Build history of the part. All positions in model axes, mm. A direction names the side the tool comes from. Round coordinates to 2 decimals unless told otherwise and drop trailing zeros. Loops run counter-clockwise (first coordinate to the right, second up) from the corner with the lowest first, then second, coordinate; pieces in that order, holes last. Notation, with made-up numbers: M 2.5,43 L 11.5,43 A33 ccw 11.5,71 Z; hole C -26.75,-0.75 d2. An arc over 180 degrees is marked long. Write each question's results on one line, items separated by ' | '. Start each with the question number.
```python
from build123d import *

# Parameters (mm, degrees)
F0_R     = 63.5
F0_R_2   = 6.35
F1_DEPTH = 12.7
F0_W     = 12.7
F0_H     = 50.8
F2_DEPTH = 127
F0_W_2   = 25.4
F3_DEPTH = 25.4
F4_R     = 9.525
F5_DEPTH = 254
F6_R     = 3.81


with BuildPart() as f1:
    # F0 (on Front) → F1 (new body)
    with BuildSketch(Plane.XZ):
        Circle(F0_R)
        with Locations((0, -44.45)):
            Circle(F0_R_2, mode=Mode.SUBTRACT)
        with Locations((-44.45, 0)):
            Circle(F0_R_2, mode=Mode.SUBTRACT)
        Polygon((-25.4, -25.4), (-25.4, 25.4), (-12.7, 25.4), (12.7, 25.4), (25.4, 25.4), (25.4, -25.4), (12.7, -25.4), (-12.7, -25.4), align=None, mode=Mode.SUBTRACT)
        with Locations((44.45, 0)):
            Circle(F0_R_2, mode=Mode.SUBTRACT)
        with Locations((0, 44.45)):
            Circle(F0_R_2, mode=Mode.SUBTRACT)
    extrude(amount=F1_DEPTH)

    # F0 (on Front) → F2 (join)
    with BuildSketch(Plane.XZ):
        with Locations((-19.05, 0)):
            Rectangle(F0_W, F0_H)
        with Locations((19.05, 0)):
            Rectangle(F0_W, F0_H)
    extrude(amount=F2_DEPTH)

    # F0 (on Front) → F3 (join)
    with BuildSketch(Plane.XZ):
        Rectangle(F0_W_2, F0_H)
    extrude(amount=F3_DEPTH)

    # F4 (on face) → F5 (cut)
    with BuildSketch(Plane.YZ.offset(25.4)):
        with BuildLine():
            Line((-127, -25.4), (-63.5, -25.4))
            ThreePointArc((-63.5, -25.4), (-88.9, 0), (-63.5, 25.4))
            Line((-63.5, 25.4), (-127, 25.4))
            Line((-127, 25.4), (-127, -25.4))
        make_face()
        with Locations((-63.5, 0)):
            Circle(F4_R)
    extrude(amount=-F5_DEPTH, mode=Mode.SUBTRACT)

    # F6
    f6_edges = [f1.edges().sort_by_distance(p)[0] for p in [
        (0, -12.7, 25.4),
        (25.4, -12.7, 0),
        (0, -12.7, -25.4),
        (-25.4, -12.7, 0),
    ]]
    fillet(f6_edges, radius=F6_R)


solid = f1.part
```
Item 1: Saw through at C-C, the plane z = -44.45. Give the cut face in (x, y), then the cut area to 3 significant figures.
Item 2: Saw through at A-A, the plane x = 0. Give the cut face in (y, z).
Item 3: Saw through at B-B, the plane z = 0. State how many separate pieces and enclosed holes the cut face has, then the cut area to 3 significant figures.
Item 4: Drill centre lines: line 1 along X through (y, z) = (-31.5, 9.5); line 2 along Z through (x, y) = (-16, -63); line 3 along Y through (x, z) = (23, 32). Where is each one in solid material? Low to high. Write a range as [from, to].
Item 5: Tool access for faces 1 (the flat face through (25.4, -52, 0)), 2 (the flat face through (0, -24, 25.4)), 3 (the flat face through (41, -12.7, -13)): list every direction of +Z, -Z, +X, -X, +Y, -Y with a clear straight run to the whole face (end or side of a thin tool).
Item 6: Mould opens along X. For faces 4 (the cylindrical face through (0.409, -13.786, 26.546)), 5 (the cylindrical face through (-0.827, -6.261, 50.746)), 6 (the cylindrical face through (26.546, -13.786, -0.409)), 7 (the flat face through (-25.4, -52, 0)) say: released by +X, released by -X, zero draft, split by the parting line, or undercut.
Item 7: Saw through at D-D, the plane y = -67. Give the cut face in (x, z), then the cut area to 3 significant figures.
Item 8: Drop flat-ended pins along their axis: pin 1 (25 mm diameter, centred on y = -63.5, z = 0, fed in from +X); pin 2 (10 mm diameter, centred on x = -44.45, z = 0, fed in from -Y); pin 3 (10 mm diameter, centred on x = -38.5, z = 22, fed in from -Y); pin 4 (14 mm diameter, centred on x = 1, y = -31, fed in from +Z). Give the stop position or say it passes through.
Working result:
1) outline: M -45.35,-12.7 L -6.35,-12.7 L -6.35,0 L -45.35,0 Z; M 6.35,-12.7 L 45.35,-12.7 L 45.35,0 L 6.35,0 Z | area: 991 mm²
2) outline: M -25.4,-25.4 L -16.51,-25.4 A3.81 cw -12.7,-29.21 L -12.7,-38.1 L 0,-38.1 L 0,38.1 L -12.7,38.1 L -12.7,29.21 A3.81 cw -16.51,25.4 L -25.4,25.4 Z; M -12.7,-63.5 L 0,-63.5 L 0,-50.8 L -12.7,-50.8 Z; M -12.7,50.8 L 0,50.8 L 0,63.5 L -12.7,63.5 Z
3) separate pieces: 5 | enclosed holes: 0 | area: 3,070 mm²
4) line 1: x = [-25.4, -12.7], [12.7, 25.4] | line 2: z = [-25.4, -9.51], [9.51, 25.4] | line 3: y = [-12.7, 0]
5) face 1: +Z, -Z, +X, -Y | face 2: +Z, +X, -X, -Y | face 3: -Y
6) face 4: zero draft | face 5: undercut | face 6: released by +X | face 7: released by -X
7) outline: M -25.4,-25.16 L -12.7,-25.16 L -12.7,-8.86 L -25.4,-8.86 Z; M -25.4,8.86 L -12.7,8.86 L -12.7,25.16 L -25.4,25.16 Z; M 12.7,-25.16 L 25.4,-25.16 L 25.4,-8.86 L 12.7,-8.86 Z; M 12.7,8.86 L 25.4,8.86 L 25.4,25.16 L 12.7,25.16 Z | area: 828 mm²
8) pin 1: stops at x = 25.4 | pin 2: passes through | pin 3: stops at y = -12.7 | pin 4: stops at z = 25.4
